Build history of the part. All positions in model axes, mm. Face numbers are marked on the shaded views. A direction names the side the tool comes from. Give positions to 0.01 mm unless a question says otherwise; leave off trailing zeros. Loops run counter-clockwise (first coordinate to the right, second up) from the corner with the lowest first, then second, coordinate; pieces in that order, holes last.
1) Two-plate mould, pull along X, no slides. Class the marked faces 1, 2 and 3: +X half, -X half, draft (parallel to the pull), parting line (faces both ways), or undercut.
2) Band-saw the part on A-A on x = 7.25. List the corners of the cut face in (y, z), then the cut area to 3 significant figures.
3) 3-axis set-ups, long thin cutter, end or side, ignore diameter. For the marked faces 4, 5 and 6: which of +Z, -Z, +X, -X, +Y, -Y reach the whole face in a straight line?
4) Band-saw the part on D-D on z = 4. State how many separate pieces and enclosed holes the cut face has, then the cut area to 3 significant figures.
5) Flat gauge pins, fed straight in: P1, Ø6, axis at y = 9, z = 3.5, coming from the -X side; P2, Ø3, axis at x = 8, y = 18, coming from the +Z side; P3, Ø4, axis at x = 5.5, z = 4.5, coming from the +Y side; P4, Ø4, axis at x = 2, y = 7, coming from the +Z side. Where does each tip first touch, or does it go through?
6) Band-saw the part on B-B on z = 10.5. List the corners of the cut face in (x, y).
7) Band-saw the part on C-C on y = 10. List the corners of the cut face in (x, z).
8) Wall check: line 1 (Y direction, x = 0, z = 2); line 2 (Z direction, x = 3, y = 5); line 3 (Y direction, x = 0, z = 4). Give the ranges that are in metal, low to high.
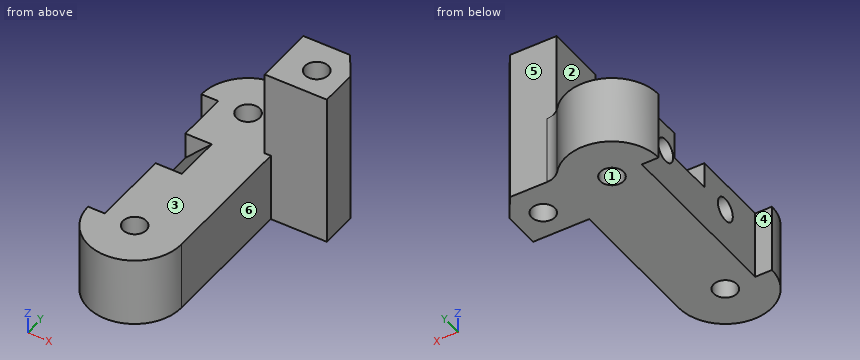
```python
from build123d import *

# Parameters (mm, degrees)
EXTRUDE_1_DEPTH        = 7.4
EXTRUDE_2_DEPTH        = 9.2
HOLE_WIZARD_M3_1_D     = 2.5
HOLE_WIZARD_M3_1_DEPTH = 6.5
HOLE_WIZARD_M3_1_TIP   = 0.751075774
HOLE_WIZARD_M3_3_D     = 2.5
FILLET_1_R             = 2
CUT_EXTRUDE_1_DEPTH    = 5
HOLE_WIZARD_M3_5_D     = 2.5


with BuildPart() as part:
    # 草图1 → 凸台-拉伸1 (new body)
    with BuildSketch(Plane.XY):
        with BuildLine():
            Line((-3.2, 19), (-3.2, 0))
            Line((-3.2, 0), (-5, 0))
            ThreePointArc((-5, 0), (0, -5), (5, 0))
            Line((5, 0), (5, 4))
            Line((5, 4), (5, 15))
            Line((5, 15), (11, 15))
            Line((11, 15), (11, 19))
            Line((11, 19), (9.333333333, 21.494438258))
            Line((9.333333333, 21.494438258), (4.333333333, 21.494438258))
            ThreePointArc((4.333333333, 21.494438258), (-1.290994449, 23.830458915), (-5, 19))
            Line((-5, 19), (-3.2, 19))
        make_face()
    extrude(amount=EXTRUDE_1_DEPTH)

    # 草图2 → 凸台-拉伸2 (add)
    with BuildSketch(Plane.XY.offset(7.4)):
        Polygon((11, 19), (9.333333333, 21.494438258), (4.333333333, 21.494438258), (4.333333333, 15), (5, 15), (11, 15), align=None)
    extrude(amount=EXTRUDE_2_DEPTH)

    # M3 螺纹孔1
    with Locations(Plane(origin=(-3.2, 15, 4.4), x_dir=(0, -1, 0), z_dir=(-1, 0, 0))):
        with Locations((0, 0), (10, 0)):
            Hole(HOLE_WIZARD_M3_1_D / 2, depth=HOLE_WIZARD_M3_1_DEPTH)
            with Locations((0, 0, -(HOLE_WIZARD_M3_1_DEPTH + HOLE_WIZARD_M3_1_TIP / 2))):  # 118° drill point
                Cone(0, HOLE_WIZARD_M3_1_D / 2, HOLE_WIZARD_M3_1_TIP, mode=Mode.SUBTRACT)

    # M3 螺纹孔3 (through all)
    with Locations(Plane.XY.offset(7.4)):
        with Locations((0, 0), (0, 19)):
            Hole(HOLE_WIZARD_M3_3_D / 2)

    # 圆角1
    fillet_1_edges = [part.edges().sort_by_distance(p)[0] for p in [
        (4.333333333, 21.494438258, 3.7),
    ]]
    fillet(fillet_1_edges, radius=FILLET_1_R)

    # 草图10 → 切除-拉伸1 (cut)
    with BuildSketch(Plane(origin=(0, 13.5, 0), x_dir=(1, 0, 0), z_dir=(0, 1, 0))):
        Polygon((-3.2, -7.4), (-0.371572875, -7.4), (-3.2, -4.571572875), align=None)
    extrude(amount=-CUT_EXTRUDE_1_DEPTH, mode=Mode.SUBTRACT)

    # M3 螺纹孔5 (through all)
    with Locations(Plane(origin=(8, 18, 16.6), x_dir=(1, 0, 0), z_dir=(0, 0, 1))):
        with Locations((0, 0)):
            Hole(HOLE_WIZARD_M3_5_D / 2)


solid = part.part
```
Findings below:
1. face 1: undercut
1. face 2: -X half
1. face 3: draft
2. outline: (15, 0) - (17, 0) - (17, 16.6) - (15, 16.6) - close; (19, 0) - (21.49, 0) - (21.49, 16.6) - (19, 16.6) - close
2. area: 74.6 mm2
3. face 4: +Z, -Z, -X
3. face 5: +Z, +X, +Y
3. face 6: +Z, -Z, +X, -Y
4. separate pieces: 1
4. enclosed holes: 3
4. area: 225 mm2
5. P1: stops at x = -3.2
5. P2: stops at z = 16.6
5. P3: stops at y = 22.57
5. P4: stops at z = 7.4
6. outline: (4.33, 15) - (11, 15) - (11, 19) - (9.33, 21.49) - (4.33, 21.49) - close; hole circle Ø2.5 at (8, 18)
7. outline: (-3.2, 0) - (5, 0) - (5, 7.4) - (-0.37, 7.4) - (-3.2, 4.57) - close
8. line 1: y = -5 to -1.25, 1.25 to 17.75, 20.25 to 24
8. line 2: z = 0 to 3.15, 5.65 to 7.4
8. line 3: y = -5 to -1.25, 1.25 to 3.82, 6.18 to 13.82, 16.18 to 17.75, 20.25 to 24
